from build123d import *

# Parameters (mm, degrees)
F1_DEPTH = 3


with BuildPart() as f1:
    # F0 (on Top) → F1 (new body)
    with BuildSketch(Plane.XY):
        Polygon((-2.297005, -1.893192), (-6.368706, -3.686192), (-4.090005, -5.9655), (4.069995, -5.9655), (6.348696, -3.686192), (2.276995, -1.893192), align=None)
        Polygon((6.348696, -3.686192), (6.348696, 4.473808), (2.276995, 2.680808), (2.276995, -1.893192), align=None)
        Polygon((-2.297005, 2.680808), (-6.368706, 4.473808), (-6.368706, -3.686192), (-2.297005, -1.893192), align=None)
        Polygon((4.069995, 6.753117), (-4.090005, 6.753117), (-6.368706, 4.473808), (-2.297005, 2.680808), (2.276995, 2.680808), (6.348696, 4.473808), align=None)
    extrude(amount=F1_DEPTH)


solid = f1.part
Verification items for the finished model (mm, model axes). A direction names the side the tool comes from. Give positions to 0.01 mm unless a question says otherwise; leave off trailing zeros. Loops run counter-clockwise (first coordinate to the right, second up) from the corner with the lowest first, then second, coordinate; pieces in that order, holes last. Notation, with made-up numbers: (16, -10.5) - (55, -10.5) arc R19 cw to (55, 14.5) - close; hole circle Ø10 at (50.25, 70). An arc over 180 degrees is marked (long way). Write each question's results on one line, items separated by ' | '.
1) Sectioned sample at B-B on z = 1.35. Record the boundary of the cut face in (x, y), plus the area to 3 significant figures.
Solution:
outline: (-6.37, -3.69) - (-4.09, -5.97) - (4.07, -5.97) - (6.35, -3.69) - (6.35, 4.47) - (4.07, 6.75) - (-4.09, 6.75) - (-6.37, 4.47) - close; hole (-2.3, -1.89) - (2.28, -1.89) - (2.28, 2.68) - (-2.3, 2.68) - close | area: 130 mm2
2) Sectioned sample at D-D on x = 4.5. Record the boundary of the cut face in (y, z).
Solution:
outline: (-5.54, 0) - (6.32, 0) - (6.32, 3) - (-5.54, 3) - close
3) Sectioned sample at C-C on y = 2.5. Record the boundary of the cut face in (x, z), plus the area to 3 significant figures.
Solution:
outline: (-6.37, 0) - (-2.3, 0) - (-2.3, 3) - (-6.37, 3) - close; (2.28, 0) - (6.35, 0) - (6.35, 3) - (2.28, 3) - close | area: 24.4 mm2
4) Sectioned sample at A-A on x = 0.5. Record the boundary of the cut face in (y, z), plus the area to 3 significant figures.
Solution:
outline: (-5.97, 0) - (-1.89, 0) - (-1.89, 3) - (-5.97, 3) - close; (2.68, 0) - (6.75, 0) - (6.75, 3) - (2.68, 3) - close | area: 24.4 mm2
5) Mould release check, pull along Y, two halves, no side actions. Record for faces 1 (the flat face through (-3, 0, 0)), 2 (the flat face through (0, 6.753, 1)), 3 (the flat face through (0, 2.681, 1)): pulls with the +Y half, pulls with the -Y half, needs draft (parallel to the pull), parting line crosses it, or undercut.
Solution:
face 1: needs draft | face 2: pulls with the +Y half | face 3: undercut
6) Material ranges on L1, parallel to X at y = 0.25, z = 2; L2, parallel to Y at x = 1.25, z = 0.25; L3, parallel to X at y = 5, z = 0.4, recorded low to high. Write a range as from..to.
Solution:
L1: -6.37..-2.3, 2.28..6.35 | L2: -5.97..-1.89, 2.68..6.75 | L3: -5.84..5.82
7) Depth check by flat-ended pin: P1, Ø4, axis at x = 2, y = 5, coming from the -Z side. Enter the tip coordinate at first touch or a pass-through.
Solution:
P1: z = 0
8) Tool access check on faces 4 (the flat face through (2.277, 0, 1)), 5 (the flat face through (6.349, 0, 1)). Record the directions out of +Z, -Z, +X, -X, +Y, -Y that give a thin tool (end or side, any length) a straight path to the whole face; none if there is none.
Solution:
face 4: +Z, -Z | face 5: +Z, -Z, +X, +Y, -Y
